Geometry: final body of the model. Coordinates: model frame, mm. Face numbers are marked on the shaded views. A direction names the side the tool comes from. Give positions to 0.01 mm unless a question says otherwise; leave off trailing zeros. Write each loop counter-clockwise with the first axis right and the second up, starting at its lowest first coordinate (ties: lowest second). Pieces come first, ordered by that corner, then holes. Notation, with made-up numbers: (-10, 73) -> (10, 73) arc R26 cw to (10, 91) -> close; hole circle Ø11 at (13, 6). An arc over 180 degrees is marked (long way). Use CSV: the item, a comma, the result in double quotes. Start each with the question number.
1) Draft query along X for the marked faces 1, 2, 3 and 4. Return one class per face: pulls with the +X half, pulls with the -X half, needs draft (parallel to the pull), parting line crosses it, or undercut.
2) Material intervals for line 1 (X direction, y = -14, z = 5.5); line 2 (Y direction, x = 10.5, z = 13.5); line 3 (Y direction, x = 8, z = 21.25), sorted ascending. Write a range as [from, to].
3) Section A-A (y = 0). Output: boundary loops of the cut face in (x, z).
4) Set-up query: the marked faces 5, 6, 7, 8 and 9. Return all of +Z, -Z, +X, -X, +Y, -Y with unobstructed straight access to the full face (end or side cutting, diameter ignored); none if empty.
5) Section C-C (z = 8.5). Output: boundary loops of the cut face in (x, y), plus the area to 3 significant figures.
6) Contact query for flat-ended pins moving along their axis: P1, Ø12, axis at x = -6, y = -22.5, coming from the -Z side; P2, Ø1.5, axis at y = 14, z = 12.5, coming from the +X side; P3, Ø4, axis at y = 1.5, z = 12, coming from the -X side; P4, Ø5, axis at y = -1, z = 5, coming from the +X side. Output: stop coordinate, or through.
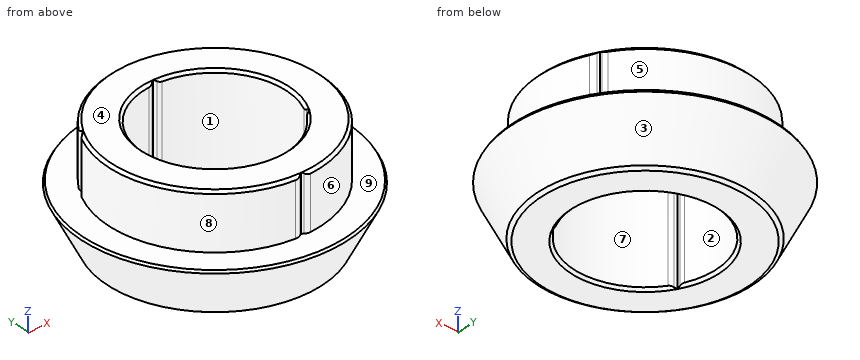
Autodesk Inventor part; units mm, degrees
ref_plane "YZ Plane" through (0, 0, 0) normal (1, 0, 0) x (0, 1, 0)
ref_plane "XZ Plane" through (0, 0, 0) normal (0, 1, 0) x (-1, 0, 0)
ref_plane "XY Plane" through (0, 0, 0) normal (0, 0, 1) x (1, 0, 0)
sketch "Sketch1" plane through (0, 0, 0) normal (0, 0, 1) x (1, 0, 0)
  circle A0 centre (0, 0) radius 15.95
  circle A1 centre (0, 0) radius 23.7
  dimension "d0" = 47.4
  dimension "d1" = 31.9
extrude "Extrusion1" add sketch "Sketch1" along normal blind 25
sketch "Sketch2" plane through (0, 0, 0) normal (1, 0, 0) x (0, 1, 0)
  line L0 (23.7, 0) -> (23.7, 25)
  line L1 (23.7, 0) -> (30, 12.5)
  line L2 (30, 12.5) -> (23.7, 12.5)
  line L3 (0, 0) -> (0, 25)
  line L4 (23.7, 25) -> (-23.7, 25)
  point P0 (0, 12.5)
  dimension "d4" = 12.5
  dimension "d5" = 60
revolve "Revolution1" add sketch "Sketch2" angle 360 about axis through (0, 0, 0) along (0, 0, 1)
sketch "Sketch3" plane through (0, 0, 25) normal (0, 0, 1) x (1, 0, 0)
  circle A0 centre (0, 0) radius 15.95
  circle A1 centre (0, 0) radius 15.95
  line L0 (-1, 15.9186) -> (0, 16.5819)
  line L1 (0, 16.5819) -> (1, 15.9186)
  line L2 (-1, 15.9186) -> (1, 15.9186)
  circle A2 centre (0, 0) radius 23.7
  line L3 (20.0065, 12.7055) -> (19.9321, 11.5078)
  line L4 (19.9321, 11.5078) -> (21.0065, 10.9734)
  line L5 (20.0065, 12.7055) -> (21.0065, 10.9734)
  line L6 (20.5065, 11.8394) -> (0, 0) construction
  line L7 (0, 0) -> (0, 16.5819) construction
  dimension "d11" = 1.2
  dimension "d12" = 2
  dimension "d16" = 1.2
  dimension "d17" = 2
  dimension "d26" = 60
extrude "Extrusion2" cut sketch "Sketch3" against normal through all contours L2 A0 | A0 L0 L1 picked at (-0.1112, 15.9279)
extrude "Extrusion3" cut sketch "Sketch3" against normal up to surface (12.5 mm away) contours L5 A2 | L4 L3 L5
pattern_circular "Circular Pattern1" count 3 over 360 about axis through (0, 0, 0) along (0, 0, 1) of "Extrusion3"
pattern_circular "Circular Pattern2" count 3 over 360 about axis through (0, 0, 0) along (0, 0, 1) of "Extrusion2"
chamfer "Chamfer1" distance 0.6 angle 45 11 edges at (-13.8131, 7.975, 0) (0, -15.95, 0) (13.8131, 7.975, 0) (0, -23.7, 0) (0, -30, 12.5) (20.5248, -11.85, 25) (0, 23.7, 25) (-20.5248, -11.85, 25) (-13.8131, 7.975, 25) (0, -15.95, 25) (13.8131, 7.975, 25)
fillet "Fillet1" radius 2 12 edges at (-1, 15.9186, 12.5) (1, 15.9186, 12.5) (20.0065, 12.7055, 18.45) (21.0065, 10.9734, 18.45) (-1, -23.6789, 18.45) (1, -23.6789, 18.45) (-20.0065, 12.7055, 18.45) (-21.0065, 10.9734, 18.45) (-13.2859, -8.8253, 12.5) (-14.2859, -7.0933, 12.5) (13.2859, -8.8253, 12.5) (14.2859, -7.0933, 12.5)
properties part number "TouptekAdapterCylinder" material "ABS Plastic"
Answers follow:
1,face 1,"undercut"
1,face 2,"undercut"
1,face 3,"parting line crosses it"
1,face 4,"needs draft"
2,line 1,"x = [-22.47, -7.64], [7.64, 22.47]"
2,line 2,"y = [-21.25, -12.01], [12.01, 21.25]"
2,line 3,"y = [-22.31, -13.8], [13.8, 22.31]"
3,outline,"(-29.73, 11.96) -> (-23.97, 0.54) -> (-23.1, 0) -> (-16.55, 0) -> (-15.95, 0.6) -> (-15.95, 24.4) -> (-16.55, 25) -> (-23.1, 25) -> (-23.7, 24.4) -> (-23.7, 12.5) -> (-29.4, 12.5) -> close; (15.95, 0.6) -> (16.55, 0) -> (23.1, 0) -> (23.97, 0.54) -> (29.73, 11.96) -> (29.4, 12.5) -> (23.7, 12.5) -> (23.7, 24.4) -> (23.1, 25) -> (16.55, 25) -> (15.95, 24.4) -> close"
4,face 5,"+Z, +Y"
4,face 6,"+Z, +X"
4,face 7,"+Z, -Z"
4,face 8,"+Z, -X"
4,face 9,"+Z"
5,outline,"circle Ø55.97 at (0, 0); hole (-14.5, -6.65) arc R2 cw to (-14.32, -7.61) -> (-14.36, -8.29) -> (-13.75, -8.59) arc R2 cw to (-13.01, -9.23) arc R15.95 ccw to (13.01, -9.23) arc R2 cw to (13.75, -8.59) -> (14.36, -8.29) -> (14.32, -7.61) arc R2 cw to (14.5, -6.65) arc R15.95 ccw to (1.49, 15.88) arc R2 cw to (0.57, 16.21) -> (0, 16.58) -> (-0.57, 16.21) arc R2 cw to (-1.49, 15.88) arc R15.95 ccw to start"
5,area,"1,660 mm^2"
6,P1,"stops at z = 0"
6,P2,"stops at x = 26.5"
6,P3,"stops at x = -29.73"
6,P4,"stops at x = 27.46"
